Read the model definition and answer for the solid it produces. Units are mm, in the model's axes. A direction names the side the tool comes from. Coordinates: 2 decimals unless noted, no trailing zeros. Write each loop counter-clockwise with the first axis right and the second up, starting at its lowest first coordinate (ties: lowest second). Pieces come first, ordered by that corner, then holes. Notation, with made-up numbers: (76, 12) -> (126, 12) arc R13 ccw to (126, 34) -> close; hole circle Ø3 at (5.5, 1). An arc over 180 degrees is marked (long way). One line per item, written item: value. Start each with the question number.
1. Find section C-C, the plane z = -19.83. Write down the section's boundary in (x, y), and give its area (3 significant figures).
2. Find section B-B, the plane y = 21.6. Write down the section's boundary in (x, z).
3. Find section D-D, the plane z = -114. State how many separate pieces and enclosed holes the cut face has, and give its area (3 significant figures).
4. Find section A-A, the plane x = -25.1. Write down the section's boundary in (y, z), and give its area (3 significant figures).
5. For a pull along X with two mould halves and no side action, classify faces 1 (the flat face through (-26, 22, -125)), 2 (the cylindrical face through (-39.3, 23.6, -7.2)) as pulls with the +X half, pulls with the -X half, needs draft (parallel to the pull), parting line crosses it, or undercut.
6. Given P1, Ø4, axis at x = -9.5, z = -52.5, coming from the -Y side; P2, Ø4, axis at x = -10.6, z = -42.2, coming from the +Y side; P3, Ø1.5, axis at y = 24, z = -44.5, coming from the -X side, each flat-ended and moving along its own axis, determine where each tip first touches the part or whether it passes through.
7. For faces 3 (the flat face through (-47.5, 22, -61)), 4 (the cylindrical face through (-12, 24.1, -9.8)), 5 (the flat face through (-39, 24.1, -115)), determine the directions among +Z, -Z, +X, -X, +Y, -Y from which every point of the face is accessible in a straight line to the end or side of a thin tool.
8. Consider line 1 along Z through (x, y) = (-25.5, 22.9); line 2 along X through (y, z) = (22, -83); line 3 along Z through (x, y) = (-25.5, 23.7). Determine where each line is inside the solid, lowest interval first.
Autodesk Inventor part; units mm, degrees
ref_plane "Work Plane2 - PCB Vertical" through (0, 0, -62.5) normal (0, 0, 1) x (1, 0, 0)
ref_plane "Work Plane6 - Fond creusé" through (0, 17, 0) normal (0, 1, 0) x (-1, 0, 0)
ref_plane "Work Plane11 - Haut capteurs shields" through (0, 23.1, 0) normal (0, 1, 0) x (-1, 0, 0)
sketch "Sketch1" plane through (0, 0, 0) normal (0, 1, 0) x (-1, 0, 0)
  line L0 (2, 0) -> (102, 0)
  line L1 (104, -2) -> (104, -123)
  line L2 (102, -125) -> (2, -125)
  line L3 (0, -123) -> (0, -2)
  arc A0 (104, -2) -> (102, 0) centre (102, -2) ccw
  arc A1 (102, -125) -> (104, -123) centre (102, -123) ccw
  arc A2 (0, -123) -> (2, -125) centre (2, -123) ccw
  arc A3 (2, 0) -> (0, -2) centre (2, -2) ccw
  point P0 (0, 0)
  point P1 (104, -125)
  point P2 (0, -125)
  dimension "d0" = 104
  dimension "d1" = 125
  dimension "d2" = 2
  dimension "d3" = 2
extrude "Boîte extérieure" [suppressed]
fillet "Fillet1-Boîte extérieure" [suppressed]
ref_plane "Work Plane2 - PCB Vertical" through (0, 0, -62.5) normal (0, 0, 1) x (1, 0, 0)
ref_plane "Work Plane4 - Surface extérieure capteurs" through (0, 20.1, 0) normal (0, 1, 0) x (-1, 0, 0)
ref_plane "Work Plane6 - Fond creusé" through (0, 17, 0) normal (0, 1, 0) x (-1, 0, 0)
sketch "Sketch26" plane through (0, 20.1, 0) normal (0, 1, 0) x (-1, 0, 0)
  line L0 (16, -121) -> (36, -121)
  line L1 (47, -110) -> (47, -13)
  line L2 (36, -2) -> (16, -2)
  line L3 (5, -13) -> (5, -110)
  arc A0 (5, -110) -> (16, -121) centre (16, -110) ccw
  arc A1 (36, -121) -> (47, -110) centre (36, -110) ccw
  arc A2 (47, -13) -> (36, -2) centre (36, -13) ccw
  arc A3 (16, -2) -> (5, -13) centre (16, -13) ccw
  line L4 (0, -2) -> (0, -123)
  line L5 (0, -2) -> (0, -123)
  line L6 (104, -123) -> (104, -2)
  line L7 (2, -125) -> (102, -125)
  point P0 (0, 0)
  point P1 (47, -2)
  point P2 (47, -121)
  point P3 (5, -2)
  dimension "d158" = 42
  dimension "d159" = 119
  dimension "d160" = 11
  dimension "d161" = 5
  dimension "d186" = 4
extrude "Centreur Echantillonnage actif" [suppressed]
sketch "Sketch 22" plane through (0, 17, 0) normal (0, 1, 0) x (-1, 0, 0)
  circle A0 centre (25.1, -19.83) radius 16.5
  line L0 (99, -5) -> (99, -120)
  line L1 (9, -5) -> (99, -5)
  circle A1 centre (25.1, -47.135) radius 10.5
  circle A2 centre (25.1, -72.535) radius 10.5
  circle A3 centre (25.1, -99.84) radius 16.5
  line L2 (102, 0) -> (2, 0)
  line L3 (0, -2) -> (0, -123)
  line L4 (2, -125) -> (102, -125)
  point P0 (0, 0)
  point P1 (99, -12.0721)
  point P2 (99, -58.79)
  point P3 (16.07, -5)
  point P4 (91.93, -5)
  dimension "d124" = 33
  dimension "d126" = 14.83
  dimension "d140" = 21
  dimension "d141" = 27.305
  dimension "d142" = 21
  dimension "d143" = 25.4
  dimension "d144" = 33
  dimension "d145" = 27.305
  dimension "d196" = 73.9
  dimension "d258" = 19.83
  dimension "d259" = 25.1
  dimension "d260" = 25.16
extrude "Sensor A/Miniature or Sensoric" [suppressed]
sketch "Sketch35" plane through (0, 20.1, 0) normal (0, 1, 0) x (-1, 0, 0)
  circle A0 centre (40.5, -114) radius 1
  line L0 (47, -110) -> (47, -13)
  line L1 (16, -121) -> (36, -121)
  point P0 (0, 0)
  dimension "d235" = 2
  dimension "d244" = 6.5
  dimension "d245" = 7
extrude "Vis Centreur Chapeau" [suppressed]
pattern_linear "Rectangular Pattern3" [suppressed]
ref_plane "Work Plane10 - Chapeau ext." through (0, 25.1, 0) normal (0, 1, 0) x (-1, 0, 0)
sketch "Sketch36" plane through (0, 25.1, 0) normal (0, 1, 0) x (-1, 0, 0)
  line L0 (102, -125) -> (2, -125)
  line L1 (102, 0) -> (2, 0)
  line L2 (2.8, -125) -> (49.2, -125)
  line L3 (49.2, -125) -> (49.2, 0)
  line L4 (49.2, 0) -> (2.8, 0)
  line L5 (2.8, 0) -> (2.8, -125)
  line L6 (47, -110) -> (47, -13)
  point P0 (0, 0)
  dimension "d247" = 46.4
  dimension "d252" = 125
extrude "Chapeau" add sketch "Sketch36" against normal blind 4.9
fillet "Fillet10" radius 2 8 edges at (-49.2, 25.1, -62.5) (-26, 25.1, -125) (-49.2, 22.65, -125) (-2.8, 22.65, -125) (-2.8, 25.1, -62.5) (-2.8, 22.65, 0) (-26, 25.1, 0) (-49.2, 22.65, 0)
ref_plane "Work Plane11 - Haut capteurs shields" through (0, 23.1, 0) normal (0, 1, 0) x (-1, 0, 0)
sketch "Sketch37" plane through (0, 23.1, 0) normal (0, 1, 0) x (-1, 0, 0)
  line L0 (14.5, -1.5) -> (37.5, -1.5)
  line L1 (47.5, -11.5) -> (47.5, -111.5)
  line L2 (37.5, -121.5) -> (14.5, -121.5)
  line L3 (4.5, -111.5) -> (4.5, -11.5)
  line L4 (4.8, 0) -> (47.2, 0)
  line L5 (2.8, -123) -> (2.8, -2)
  line L6 (47.2, -125) -> (4.8, -125)
  arc A0 (4.5, -111.5) -> (14.5, -121.5) centre (14.5, -111.5) ccw
  arc A1 (37.5, -121.5) -> (47.5, -111.5) centre (37.5, -111.5) ccw
  arc A2 (47.5, -11.5) -> (37.5, -1.5) centre (37.5, -11.5) ccw
  arc A3 (14.5, -1.5) -> (4.5, -11.5) centre (14.5, -11.5) ccw
  point P0 (0, 0)
  point P1 (4.5, -1.5)
  point P2 (47.5, -121.5)
  point P3 (47.5, -1.5)
  point P4 (4.5, -121.5)
  dimension "d254" = 43
  dimension "d255" = 120
  dimension "d257" = 1.7
  dimension "d263" = 3.5
  dimension "d264" = 10
extrude "Creusement interne pour passage Centreur" cut sketch "Sketch37" against normal blind 2.9
sketch "Sketch41" plane through (0, 25.1, 0) normal (0, 1, 0) x (-1, 0, 0)
  circle A0 centre (40.5, -114) radius 1.5
  point P0 (0, 0)
  dimension "d276" = 3
extrude "Alesage de vissage chapeau" cut sketch "Sketch41" against normal blind 2
sketch "Sketch38" plane through (0, 23.1, 0) normal (0, 1, 0) x (-1, 0, 0)
  line L0 (47.2, -125) -> (4.8, -125)
  line L1 (4.8, 0) -> (47.2, 0)
  circle A0 centre (25.1, -97.935) radius 8.25
  circle A1 centre (25.1, -72.535) radius 8.25
  circle A2 centre (25.1, -47.135) radius 8.25
  point P0 (0, 0)
  point P1 (25.1, -99.84)
  point P2 (25.1, -19.83)
  point P3 (25.1, -21.735)
  dimension "d265" = 25.16
  dimension "d266" = 27.305
  dimension "d267" = 25.4
  dimension "d268" = 27.305
  dimension "d269" = 19.83
  dimension "d270" = 27.065
  dimension "d271" = 25.4
  dimension "d272" = 25.4
  dimension "d273" = 21.735
  dimension "d300" = 16.5
  dimension "d301" = 16.5
  dimension "d302" = 16.5
pattern_linear "Alesages de vissages chapeau" count 2 spacing 29.9 along (1, 0, 0) count 4 spacing 35.9 along (0, 0, 1) of "Alesage de vissage chapeau"
sketch "Sketch44" plane through (0, 25.1, 0) normal (0, 1, 0) x (-1, 0, 0)
  circle A0 centre (40.5, -114) radius 3
  point P0 (0, 0)
  dimension "d291" = 6
extrude "Epaulement tête de vis" cut sketch "Sketch44" against normal blind 1
pattern_linear "Epaulements tête de vis" count 2 spacing 29.9 along (1, 0, 0) count 4 spacing -35.9 along (0, 0, -1) of "Epaulement tête de vis"
sketch "Sketch45" plane through (0, 23.1, 0) normal (0, 1, 0) x (-1, 0, 0)
  circle A0 centre (25.1, -97.935) radius 8.4
  circle A1 centre (25.1, -72.535) radius 10.5
  circle A2 centre (25.1, -47.135) radius 10.5
  circle A3 centre (25.1, -19.83) radius 16.5
  circle A4 centre (25.1, -99.84) radius 16.5
  point P0 (0, 0)
  dimension "d308" = 33
  dimension "d309" = 33
extrude "Alesages Capteurs" [suppressed]
sketch "Sketch46" plane through (0, 23.1, 0) normal (0, 1, 0) x (-1, 0, 0)
  circle A0 centre (25.1, -99.84) radius 16.5
  circle A1 centre (25.1, -19.83) radius 16.5
  point P0 (0, 0)
  dimension "d310" = 33
  dimension "d311" = 33
extrude "Extrusion40" cut sketch "Sketch46" along normal blind 2
properties part number "160409 Sensor cover B_Compact - None - None - B_Compact - R23"
Answer block:
1. outline: (-49.2, 20.2) -> (-47.5, 20.2) -> (-47.5, 23.1) -> (-41.6, 23.1) -> (-41.6, 25.1) -> (-47.2, 25.1) arc R2 ccw to (-49.2, 23.1) -> close; (-8.6, 23.1) -> (-4.5, 23.1) -> (-4.5, 20.2) -> (-2.8, 20.2) -> (-2.8, 23.1) arc R2 ccw to (-4.8, 25.1) -> (-8.6, 25.1) -> close
1. area: 34.9 mm2
2. outline: (-49.2, -123) arc R2 ccw to (-47.2, -125) -> (-4.8, -125) arc R2 ccw to (-2.8, -123) -> (-2.8, -2) arc R2 ccw to (-4.8, 0) -> (-47.2, 0) arc R2 ccw to (-49.2, -2) -> close; hole (-47.5, -111.5) arc R10 ccw to (-37.5, -121.5) -> (-14.5, -121.5) arc R10 ccw to (-4.5, -111.5) -> (-4.5, -11.5) arc R10 ccw to (-14.5, -1.5) -> (-37.5, -1.5) arc R10 ccw to (-47.5, -11.5) -> close
3. separate pieces: 4
3. enclosed holes: 0
3. area: 50.9 mm2
4. outline: (20.2, -125) -> (23.1, -125) arc R2 ccw to (25.1, -123) -> (25.1, -116.34) -> (23.1, -116.34) -> (23.1, -121.5) -> (20.2, -121.5) -> close; (20.2, -1.5) -> (23.1, -1.5) -> (23.1, -3.33) -> (25.1, -3.33) -> (25.1, -2) arc R2 ccw to (23.1, 0) -> (20.2, 0) -> close; (23.1, -83.34) -> (25.1, -83.34) -> (25.1, -36.33) -> (23.1, -36.33) -> close
4. area: 131 mm2
5. face 1: needs draft
5. face 2: undercut
6. P1: stops at y = 23.1
6. P2: stops at y = 24.1
6. P3: stops at x = -49.19
7. face 3: -Y
7. face 4: +Y, -Y
7. face 5: +Y
8. line 1: z = -125 to -121.5, -1.5 to 0
8. line 2: x = -49.2 to -47.5, -4.5 to -2.8
8. line 3: z = -124.91 to -116.34, -83.34 to -36.33, -3.33 to -0.09
